Check sheet for the modelled part. Datum: model origin and axes. Units: mm. A direction names the side the tool comes from. Give positions to 0.01 mm unless a question says otherwise; leave off trailing zeros. Write each loop counter-clockwise with the first axis right and the second up, starting at its lowest first coordinate (ties: lowest second). Pieces come first, ordered by that corner, then holes. Notation, with made-up numbers: M 28.5,-13 L 59.5,-13 A22 cw 59.5,20 Z; hole C 87,-33.5 d1. An arc over 180 degrees is marked long. Write item = value, one per line. Start each with the question number.
1) Sectioned sample at B-B, the plane z = 0. Record the cut outline in (x, y), then the cut area to 3 significant figures.
2) Scan lines: L1, parallel to Z at x = 0, y = -13.9; L2, parallel to Z at x = 0, y = -1; L3, parallel to Y at x = 13.5, z = 10.5. Record each from-to range of solid material in increasing order.
3) Draft check along Z on faces 1 (the face through (0.33, -13.986, 6.147)), 2 (the face through (-2.539, -7.395, 19.334)), 3 (the face through (17.24, 0, -7.13)). Enter one of: pulls with the +Z half, pulls with the -Z half, needs draft (parallel to the pull), parting line crosses it, or undercut.
4) Set-up check for faces 4 (the face through (-9.09, -13.99, 0.46)), 5 (the face through (4.01, -6.41, -18.06)): record each of +Z, -Z, +X, -X, +Y, -Y from which the full face is reachable in a straight line by a thin tool's end or side.
5) Sectioned sample at A-A, the plane x = 0. Record the cut outline in (y, z).
6) Sectioned sample at D-D, the plane z = 14.5. Record the cut outline in (x, y).
7) Sectioned sample at C-C, the plane y = -9.75. Record the cut outline in (x, z).
8) Gauge pin test, flat ends, axial feed: pin 1 (2.5 mm diameter, centred on x = 0, z = -7.64, fed in from -Y); pin 2 (1.5 mm diameter, centred on y = -2, z = -6, fed in from -X); pin 3 (1 mm diameter, centred on x = 4, y = -1.5, fed in from -Z); pin 4 (1.5 mm diameter, centred on x = 2.5, y = -11, fed in from -Z). Record the tip position at first contact, or that the pin passes through.
from build123d import *

# Parameters (mm, degrees)
F0_R     = 19.5
F1_DEPTH = 15
F2_R     = 18.5
F3_DEPTH = 13
F4_R     = 4.5085
F4_R_2   = 1.524
F5_DEPTH = 2.001


with BuildPart() as f1:
    # F0 (on Front) → F1 (new body)
    with BuildSketch(Plane.XZ):
        Circle(F0_R)
    extrude(amount=F1_DEPTH)

    # F2 (on face) → F3 (cut)
    with BuildSketch(Plane(origin=(0, 0, 0), x_dir=(-1, 0, 0), z_dir=(0, 1, 0))):
        Circle(F2_R)
    extrude(amount=-F3_DEPTH, mode=Mode.SUBTRACT)

    # F4 (on face) → F5 (cut, through all)
    with BuildSketch(Plane(origin=(0, -13, 0), x_dir=(-1, 0, 0), z_dir=(0, 1, 0))):
        Circle(F4_R)
        with Locations((0, 7.63524)):
            Circle(F4_R_2)
        with Locations((-7.63524, 0)):
            Circle(F4_R_2)
        with Locations((0, -7.63524)):
            Circle(F4_R_2)
        with Locations((7.63524, 0)):
            Circle(F4_R_2)
    extrude(amount=-F5_DEPTH, mode=Mode.SUBTRACT)


solid = f1.part
Data:
q1.outline = M -19.5,-15 L -9.16,-15 L -9.16,-13 L -18.5,-13 L -18.5,0 L -19.5,0 Z; M -6.11,-15 L -4.51,-15 L -4.51,-13 L -6.11,-13 Z; M 4.51,-15 L 6.11,-15 L 6.11,-13 L 4.51,-13 Z; M 9.16,-15 L 19.5,-15 L 19.5,0 L 18.5,0 L 18.5,-13 L 9.16,-13 Z
q1.area = 73.8 mm2
q2.L1 = -19.5 to -9.16, -6.11 to -4.51, 4.51 to 6.11, 9.16 to 19.5
q2.L2 = -19.5 to -18.5, 18.5 to 19.5
q2.L3 = -15 to -13
q3.face_1 = undercut
q3.face_2 = parting line crosses it
q3.face_3 = needs draft
q4.face_4 = +Y, -Y
q4.face_5 = +Y
q5.outline = M -15,-19.5 L 0,-19.5 L 0,-18.5 L -13,-18.5 L -13,-9.16 L -15,-9.16 Z; M -15,-6.11 L -13,-6.11 L -13,-4.51 L -15,-4.51 Z; M -15,4.51 L -13,4.51 L -13,6.11 L -15,6.11 Z; M -15,9.16 L -13,9.16 L -13,18.5 L 0,18.5 L 0,19.5 L -15,19.5 Z
q6.outline = M -13.04,-15 L 13.04,-15 L 13.04,0 L 11.49,0 L 11.49,-13 L -11.49,-13 L -11.49,0 L -13.04,0 Z
q7.outline = C 0,0 d39; hole C 0,0 d37
q8.pin_1 = through
q8.pin_2 = -18.78
q8.pin_3 = -19.18
q8.pin_4 = -19.42
